For this review, take the finished solid that the model builds, in its own axes (mm). Face numbers are marked on the shaded views. Give positions to 0.01 mm unless a question says otherwise; leave off trailing zeros. Write each loop counter-clockwise with the first axis right and the second up, starting at its lowest first coordinate (ties: lowest second). Pieces come first, ordered by that corner, then holes. Notation, with made-up numbers: (11.5, -21) -> (39.5, -21) arc R25 ccw to (39.5, -6) -> close; hole circle Ø10 at (83.25, -12.5). An arc over 180 degrees is marked (long way). Return JSON: item names as keys, results as strings.
from build123d import *

# Parameters (mm, degrees)
F0_R     = 68.95504
F1_DEPTH = 26.416
F2_R     = 26.368041
F4_D     = 25.4


with BuildPart() as f1:
    # F0 (on Top) → F1 (new body)
    with BuildSketch(Plane.XY):
        Circle(F0_R)
    extrude(amount=F1_DEPTH)

    # F2
    f2_edges = [f1.edges().sort_by_distance(p)[0] for p in [
        (-68.95504, 0, 26.416),
    ]]
    fillet(f2_edges, radius=F2_R)

    # F4 (through all)
    with Locations(Plane(origin=(0, 0, 0), x_dir=(1, 0, 0), z_dir=(0, 0, -1))):
        with Locations((0, 0)):
            Hole(F4_D / 2)


solid = f1.part
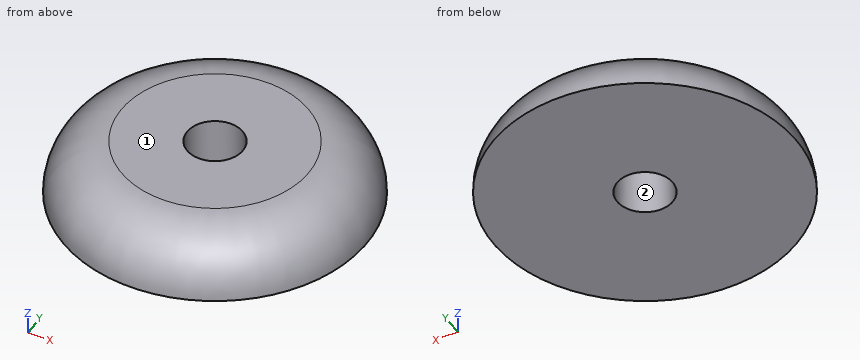
1. Add section D-D, the plane z = 14. State the section outline as (x, y) points.
Results found:
{"outline": "circle Ø129.92 at (0, 0); hole circle Ø25.4 at (0, 0)"}
2. The part is to be moulded in two halves that separate along X. For the marked faces 1 and 2, say which applies: +X half, -X half, draft (parallel to the pull), parting line (faces both ways), or undercut.
Results found:
{"face 1": "draft", "face 2": "undercut"}
3. To check wall thickness, follow probe 1 along Y at (x, z) = (5, 1.5); probe 2 along Y at (x, z) = (0, 8); probe 3 along X at (y, z) = (-9.5, 13.5). State the ranges of each line that lie inside material, in increasing order.
Results found:
{"probe 1": "y = -68.73 to -11.67, 11.67 to 68.73", "probe 2": "y = -67.73 to -12.7, 12.7 to 67.73", "probe 3": "x = -64.57 to -8.43, 8.43 to 64.57"}
4. For pin 1 (8 mm diameter, centred on y = 32, z = 7.5, fed in from -X); pin 2 (1 mm diameter, centred on y = 10, z = 7.5, fed in from +X); pin 3 (1 mm diameter, centred on y = 54, z = 4.5, fed in from -X); pin 4 (1 mm diameter, centred on x = -4.5, y = 9.5, fed in from +Z), all flat-tipped, find the tip position at first contact; note any pin that passes through.
Results found:
{"pin 1": "stops at x = -62.15", "pin 2": "stops at x = 67.3", "pin 3": "stops at x = -42.92", "pin 4": "passes through"}
5. Add section A-A, the plane x = 0. State the section outline as (y, z) points.
Results found:
{"outline": "(-68.96, 0) -> (-12.7, 0) -> (-12.7, 26.42) -> (-42.59, 26.42) arc R26.37 ccw to (-68.96, 0.05) -> close; (12.7, 0) -> (68.96, 0) -> (68.96, 0.05) arc R26.37 ccw to (42.59, 26.42) -> (12.7, 26.42) -> close"}
6. Add section C-C, the plane z = 5.5. State the section outline as (x, y) points.
Results found:
{"outline": "circle Ø136.77 at (0, 0); hole circle Ø25.4 at (0, 0)"}
